from build123d import *

# Parameters (mm, degrees)
F1_DEPTH = 12.7
F2_W     = 6.35
F2_H     = 19.05
F3_DEPTH = 6.35
F4_W     = 19.05
F4_H     = 6.35
F5_DEPTH = 6.35
F6_R     = 3.175
F7_DEPTH = 25.4
F8_DEPTH = 25.4


with BuildPart() as f1:
    # F0 (on Top) → F1 (new body)
    with BuildSketch(Plane.XY):
        Polygon((0, 19.05), (0, 0), (19.05, 0), (19.05, -6.35), (38.1, -6.35), (38.1, 19.05), align=None)
    extrude(amount=F1_DEPTH)

    # F2 (on face) → F3 (join)
    with BuildSketch(Plane(origin=(0, 0, 0), x_dir=(1, 0, 0), z_dir=(0, 0, -1))):
        with Locations((3.175, -9.525)):
            Rectangle(F2_W, F2_H)
    extrude(amount=F3_DEPTH)

    # F4 (on face) → F5 (join)
    with BuildSketch(Plane.XY.offset(12.7)):
        with Locations((28.575, 15.875)):
            Rectangle(F4_W, F4_H)
    extrude(amount=F5_DEPTH)

    # F6 (on face) → F7 (cut)
    with BuildSketch(Plane.XY.offset(12.7)):
        with Locations((28.575, 3.175)):
            Circle(F6_R)
    extrude(amount=-F7_DEPTH, mode=Mode.SUBTRACT)

    # F6 (on face) → F8 (cut)
    with BuildSketch(Plane.XY.offset(12.7)):
        with Locations((12.7, 9.525)):
            Circle(F6_R)
    extrude(amount=-F8_DEPTH, mode=Mode.SUBTRACT)


solid = f1.part
Read the model definition and answer for the solid it produces. Units are mm, in the model's axes. A direction names the side the tool comes from. Coordinates: 2 decimals unless noted, no trailing zeros. Write each loop counter-clockwise with the first axis right and the second up, starting at its lowest first coordinate (ties: lowest second). Pieces come first, ordered by that corner, then holes. Notation, with made-up numbers: (-19, 29.5) - (16, 29.5) arc R8 cw to (16, 38.5) - close; hole circle Ø4 at (-39, 40). An arc over 180 degrees is marked (long way). One line per question, with ' | ' between items.
Q1. Find section A-A, the plane x = 12.7. Write down the section's boundary in (y, z).
Result set:
outline: (0, 0) - (6.35, 0) - (6.35, 12.7) - (0, 12.7) - close; (12.7, 0) - (19.05, 0) - (19.05, 12.7) - (12.7, 12.7) - close
Q2. Find section B-B, the plane y = 7.75. Write down the section's boundary in (x, z), plus the area to 3 significant figures.
Result set:
outline: (0, -6.35) - (6.35, -6.35) - (6.35, 0) - (10.07, 0) - (10.07, 12.7) - (0, 12.7) - close; (15.33, 0) - (38.1, 0) - (38.1, 12.7) - (15.33, 12.7) - close | area: 457 mm^2
Q3. Consider L1, parallel to Y at x = 12.7, z = 4.5; L2, parallel to X at y = 3, z = 6.75; L3, parallel to X at y = -3, z = 3.5. Determine where each line is inside the solid, lowest interval first. Write a range as [from, to].
Result set:
L1: [0, 6.35], [12.7, 19.05] | L2: [0, 25.4], [31.75, 38.1] | L3: [19.05, 38.1]
Q4. Find section C-C, the plane y = 16.5. Write down the section's boundary in (x, z), plus the area to 3 significant figures.
Result set:
outline: (0, -6.35) - (6.35, -6.35) - (6.35, 0) - (38.1, 0) - (38.1, 19.05) - (19.05, 19.05) - (19.05, 12.7) - (0, 12.7) - close | area: 645 mm^2
Q5. Each of these flat-tipped pins is pushed along its axis until it touches: P1, Ø5, axis at y = -4, z = 3.5, coming from the -X side; P2, Ø8, axis at x = 23.5, y = 3.5, coming from the -Z side; P3, Ø5, axis at y = 15.5, z = 15.5, coming from the -X side. Where does it stop, or does it pass through?
Result set:
P1: x = 19.05 | P2: z = 0 | P3: x = 19.05
Q6. Determine the mould class of faces 1 (the flat face through (19.05, -3, 6)), 2 (the flat face through (19, 19.05, 6)), 3 (the cylindrical face through (26.235, 5.321, 6.439)) for opening direction Y: +Y half, -Y half, draft (parallel to the pull), parting line (faces both ways), or undercut.
Result set:
face 1: draft | face 2: +Y half | face 3: undercut
Q7. Find section D-D, the plane z = 5.5. Write down the section's boundary in (x, y) (3 decimals).
Result set:
outline: (0, 0) - (19.05, 0) - (19.05, -6.35) - (38.1, -6.35) - (38.1, 19.05) - (0, 19.05) - close; hole circle Ø6.35 at (12.7, 9.525); hole circle Ø6.35 at (28.575, 3.175)
Q8. For faces 4 (the flat face through (9, 0, 5)), 5 (the flat face through (6.35, 10, -3)), 6 (the flat face through (19.05, 16, 16)), 7 (the flat face through (0, 10, 3)), 8 (the flat face through (28, 12.7, 16)), determine the directions among +Z, -Z, +X, -X, +Y, -Y from which every point of the face is accessible in a straight line to the end or side of a thin tool.
Result set:
face 4: +Z, -Z, -X, -Y | face 5: -Z, +X, +Y, -Y | face 6: +Z, -X, +Y, -Y | face 7: +Z, -Z, -X, +Y, -Y | face 8: +Z, +X, -X, -Y
